```python
from build123d import *

# Parameters (mm, degrees)
SKETCH1_W           = 78
SKETCH1_H           = 45
SKETCH1_R           = 1.75
BOSS_EXTRUDE1_DEPTH = 3
SKETCH2_W           = 78
SKETCH2_H           = 3
BOSS_EXTRUDE2_DEPTH = 70
CUT_EXTRUDE1_DEPTH  = 101.430324106
FILLET1_R           = 5
FILLET2_R           = 10
FILLET3_R           = 3


with BuildPart() as part:
    # Sketch1 → Boss-Extrude1 (new body)
    with BuildSketch(Plane.XY):
        Rectangle(SKETCH1_W, SKETCH1_H)
        with Locations((-35, 17.5)):
            Circle(SKETCH1_R, mode=Mode.SUBTRACT)
        with Locations((35, 17.5)):
            Circle(SKETCH1_R, mode=Mode.SUBTRACT)
        with Locations((35, -17.5)):
            Circle(SKETCH1_R, mode=Mode.SUBTRACT)
        with Locations((-35, -17.5)):
            Circle(SKETCH1_R, mode=Mode.SUBTRACT)
    extrude(amount=BOSS_EXTRUDE1_DEPTH)

    # Sketch2 → Boss-Extrude2 (add)
    with BuildSketch(Plane.XZ.offset(22.5)):
        with Locations((0, 1.5)):
            Rectangle(SKETCH2_W, SKETCH2_H)
    extrude(amount=BOSS_EXTRUDE2_DEPTH)

    # Sketch3 → Cut-Extrude1 (cut, through all)
    with BuildSketch(Plane.XY.offset(3)):
        with BuildLine():
            Line((41, -36.924564207), (91.469533364, -36.924564207))
            Line((91.469533364, -36.924564207), (78.54293296, -118.649611561))
            Line((78.54293296, -118.649611561), (-67.027042434, -120.25516276))
            Line((-67.027042434, -120.25516276), (-84.509711048, -42.475126887))
            Line((-84.509711048, -42.475126887), (-81.655397805, -36.924564207))
            Line((-81.655397805, -36.924564207), (-41, -36.924564207))
            Line((-41, -36.924564207), (-41, -55.5))
            ThreePointArc((-41, -55.5), (-39.574767078, -61.537383539), (-35.6, -66.3))
            Line((-35.6, -66.3), (-27.6, -72.3))
            ThreePointArc((-27.6, -72.3), (-22.741951349, -78.120975674), (-21, -85.5))
            Line((-21, -85.5), (-21, -101))
            ThreePointArc((-21, -101), (-19.389087297, -104.889087297), (-15.5, -106.5))
            Line((-15.5, -106.5), (15.5, -106.5))
            ThreePointArc((15.5, -106.5), (19.389087297, -104.889087297), (21, -101))
            Line((21, -101), (21, -85.5))
            ThreePointArc((21, -85.5), (22.741951349, -78.120975674), (27.6, -72.3))
            Line((27.6, -72.3), (35.6, -66.3))
            ThreePointArc((35.6, -66.3), (39.574767078, -61.537383539), (41, -55.5))
            Line((41, -55.5), (41, -36.924564207))
        make_face()
    extrude(amount=-CUT_EXTRUDE1_DEPTH, mode=Mode.SUBTRACT)

    # Fillet1
    fillet1_edges = [part.edges().sort_by_distance(p)[0] for p in [
        (21, -92.5, 1.5),
        (-21, -92.5, 1.5),
    ]]
    fillet(fillet1_edges, radius=FILLET1_R)

    # Fillet2
    fillet2_edges = [part.edges().sort_by_distance(p)[0] for p in [
        (39, -62.571067812, 1.5),
        (-39, -62.571067812, 1.5),
    ]]
    fillet(fillet2_edges, radius=FILLET2_R)

    # Fillet3
    fillet3_edges = [part.edges().sort_by_distance(p)[0] for p in [
        (-39, 22.5, 1.5),
        (39, 22.5, 1.5),
    ]]
    fillet(fillet3_edges, radius=FILLET3_R)


solid = part.part
```
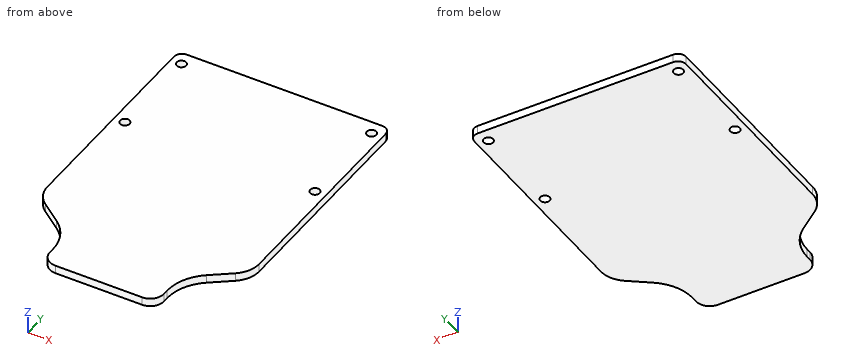
Input: part model. Units: mm. Frame: model coordinates. Give positions to 0.01 mm unless a question says otherwise; leave off trailing zeros. Order: outer loops, then holes, each group sorted by start corner. A loop starts at its lowest first (then second) coordinate and runs counter-clockwise, first axis right, second up.
1. Cut plane C-C (z = 2.05). State how many separate pieces and enclosed holes the cut face has, and give its area (3 significant figures).
Computed:
separate pieces: 1
enclosed holes: 4
area: 8,140 mm2
2. Cut plane B-B (x = 29). Return loops of the section in (y, z), and give its area (3 significant figures).
Computed:
outline: (-71.25, 0) - (22.5, 0) - (22.5, 3) - (-71.25, 3) - close
area: 281 mm2
3. Pin query (flat end, axial travel): pin 1 Ø2 at (x, y) = (-35, -17.5) entering from -Z; pin 2 Ø0.6 at (y, z) = (-86, 1.5) entering from +X. Return the tip coordinate at first contact, or that it passes through.
Computed:
pin 1: passes through
pin 2: stops at x = 21
4. Cut plane A-A (y = -17.5). Return loops of the section in (x, z), and give its area (3 significant figures).
Computed:
outline: (-39, 0) - (-36.75, 0) - (-36.75, 3) - (-39, 3) - close; (-33.25, 0) - (33.25, 0) - (33.25, 3) - (-33.25, 3) - close; (36.75, 0) - (39, 0) - (39, 3) - (36.75, 3) - close
area: 213 mm2
5. Line query: probe 1 along Y at (x, z) = (35, 1.25); probe 2 along Y at (x, z) = (-17, 2.4). Output: solid intervals per line, ascending.
Computed:
probe 1: y = -66.75 to -19.25, -15.75 to 15.75, 19.25 to 22.5
probe 2: y = -92.4 to 22.5
